Verification items for the finished model (mm, model axes). A direction names the side the tool comes from. Round coordinates to 2 decimals unless told otherwise and drop trailing zeros. Write each loop counter-clockwise with the first axis right and the second up, starting at its lowest first coordinate (ties: lowest second). Pieces come first, ordered by that corner, then holes. Notation, with made-up numbers: (86.25, -30.75) -> (136.25, -30.75) arc R8 ccw to (136.25, -26.75) -> close; hole circle Ø4 at (42.25, 25.25). An arc over 180 degrees is marked (long way). Use CSV: the item, a comma, the result in double quotes.
```python
from build123d import *

# Parameters (mm, degrees)
SKETCH3_R           = 11.125
SKETCH3_R_2         = 3.6
BOSS_EXTRUDE1_DEPTH = 8
SKETCH4_R           = 9
SKETCH4_R_2         = 3.6
BOSS_EXTRUDE3_DEPTH = 2
CUT_EXTRUDE1_REACH  = 51.5
SKETCH5_R           = 1.5
CUT_EXTRUDE2_REACH  = 51.5
SKETCH6_R           = 1.5


with BuildPart() as part:
    # Sketch3 → Boss-Extrude1 (new body)
    with BuildSketch(Plane.XY):
        Polygon((8.660254038, 15), (-8.660254038, 15), (-13.856406461, 6), (-20.784609691, 6), (-24.248711306, 0), (-20.784609691, -6), (-13.856406461, -6), (-8.660254038, -15), (8.660254038, -15), (13.856406461, -6), (20.784609691, -6), (24.248711306, 0), (20.784609691, 6), (13.856406461, 6), align=None)
        Circle(SKETCH3_R, mode=Mode.SUBTRACT)
        with Locations((17.320508076, 0)):
            Circle(SKETCH3_R_2, mode=Mode.SUBTRACT)
        with Locations((-17.320508076, 0)):
            Circle(SKETCH3_R_2, mode=Mode.SUBTRACT)
    extrude(amount=BOSS_EXTRUDE1_DEPTH)

    # Sketch4 → Boss-Extrude3 (add)
    with BuildSketch(Plane.XY.offset(8)):
        Polygon((-8.660254038, 15), (-13.856406461, 6), (-20.784609691, 6), (-24.248711306, 0), (-20.784609691, -6), (-13.856406461, -6), (-8.660254038, -15), (8.660254038, -15), (13.856406461, -6), (20.784609691, -6), (24.248711306, 0), (20.784609691, 6), (13.856406461, 6), (8.660254038, 15), align=None)
        Circle(SKETCH4_R, mode=Mode.SUBTRACT)
        with Locations((-17.320508076, 0)):
            Circle(SKETCH4_R_2, mode=Mode.SUBTRACT)
        with Locations((17.320508076, 0)):
            Circle(SKETCH4_R_2, mode=Mode.SUBTRACT)
    extrude(amount=BOSS_EXTRUDE3_DEPTH)

    # Sketch5 → Cut-Extrude1 (cut, up to next)
    with BuildSketch(Plane(origin=(-18.186533479, 10.5, 0), x_dir=(0, 0, 1), z_dir=(-0.866025404, 0.5, 0)), mode=Mode.PRIVATE) as cut_extrude1_sk1:
        with Locations((5, -8.660254038)):
            Circle(SKETCH5_R)
    cut_extrude1_tool1 = extrude(cut_extrude1_sk1.sketch, amount=-CUT_EXTRUDE1_REACH, mode=Mode.PRIVATE) & part.part
    add(cut_extrude1_tool1.solids().sort_by_distance((-22.51666, 3, 5))[0], mode=Mode.SUBTRACT)

    # Sketch6 → Cut-Extrude2 (cut, up to next)
    with BuildSketch(Plane(origin=(18.186533479, 10.5, 0), x_dir=(0, 0, -1), z_dir=(0.866025404, 0.5, 0)), mode=Mode.PRIVATE) as cut_extrude2_sk1:
        with Locations((-5, -8.660254038)):
            Circle(SKETCH6_R)
    cut_extrude2_tool1 = extrude(cut_extrude2_sk1.sketch, amount=-CUT_EXTRUDE2_REACH, mode=Mode.PRIVATE) & part.part
    add(cut_extrude2_tool1.solids().sort_by_distance((22.51666, 3, 5))[0], mode=Mode.SUBTRACT)


solid = part.part
```
Q1. Material ranges on L1, parallel to X at y = 2.5, z = 0.75; L2, parallel to Y at x = 0, z = 3.75 (3 decimals); L3, parallel to Z at x = -5, y = -9.75, recorded low to high.
Filled in:
L1,"-22.81 to -19.91, -14.73 to -10.84, 10.84 to 14.73, 19.91 to 22.81"
L2,"-15 to -11.125, 11.125 to 15"
L3,"8 to 10"
Q2. Access from +Z, -Z, +X, -X, +Y, -Y to the whole of each face (thin tool, end or side, straight path). Record for faces 1 (the cylindrical face through (-8.2, 7.52, 3.94)), 2 (the flat face through (17, -6, 5)), 3 (the flat face through (-11.295, -10.437, 4.93)), 4 (the flat face through (-17, 6, 5)).
Filled in:
face 1,"-Z"
face 2,"+Z, -Z, +X, -Y"
face 3,"+Z, -Z, -X, -Y"
face 4,"+Z, -Z, -X, +Y"
Q3. Section check A-A (x = 0). Record the cut outline in (y, z) (3 decimals).
Filled in:
outline,"(-15, 0) -> (-11.125, 0) -> (-11.125, 8) -> (-9, 8) -> (-9, 10) -> (-15, 10) -> close; (9, 8) -> (11.125, 8) -> (11.125, 0) -> (15, 0) -> (15, 10) -> (9, 10) -> close"
Q4. Section check B-B (z = 8.75). Record the cut outline in (x, y).
Filled in:
outline,"(-24.25, 0) -> (-20.78, -6) -> (-13.86, -6) -> (-8.66, -15) -> (8.66, -15) -> (13.86, -6) -> (20.78, -6) -> (24.25, 0) -> (20.78, 6) -> (13.86, 6) -> (8.66, 15) -> (-8.66, 15) -> (-13.86, 6) -> (-20.78, 6) -> close; hole circle Ø7.2 at (-17.32, 0); hole circle Ø18 at (0, 0); hole circle Ø7.2 at (17.32, 0)"
Q5. Section check C-C (y = 5). Record the cut outline in (x, z), plus the area to 3 significant figures.
Filled in:
outline,"(-21.36, 0) -> (-9.94, 0) -> (-9.94, 8) -> (-7.48, 8) -> (-7.48, 10) -> (-21.36, 10) -> close; (7.48, 8) -> (9.94, 8) -> (9.94, 0) -> (21.36, 0) -> (21.36, 10) -> (7.48, 10) -> close"
area,"238 mm²"
Q6. Mould release check, pull along Y, two halves, no side actions. Record for faces 5 (the flat face through (-22.54, -2.96, 4.93)), 6 (the flat face through (17, 6, 5)), 7 (the cylindrical face through (-1.172, 8.923, 8.986)), 8 (the flat face through (9, 7, 0)): released by +Y, released by -Y, zero draft, split by the parting line, or undercut.
Filled in:
face 5,"released by -Y"
face 6,"released by +Y"
face 7,"undercut"
face 8,"zero draft"
Q7. Go/stop test with flat-tipped pins: P1, Ø3.5, axis at x = -17, z = 7.5, coming from the +Y side; P2, Ø3.5, axis at x = 16, z = 3.5, coming from the -Y side; P3, Ø4, axis at y = -8.5, z = 5, coming from the -X side. Record where each tip stops, or that it passes through.
Filled in:
P1,"y = 6"
P2,"y = -6"
P3,"x = -13.57"
